Autodesk Inventor part; units mm, degrees
ref_plane "YZ Plane" through (0, 0, 0) normal (1, 0, 0) x (0, 1, 0)
ref_plane "XZ Plane" through (0, 0, 0) normal (0, 1, 0) x (-1, 0, 0)
ref_plane "XY Plane" through (0, 0, 0) normal (0, 0, 1) x (1, 0, 0)
sketch "Esboço1" plane through (0, 0, 0) normal (0, 1, 0) x (-1, 0, 0)
  arc A0 (-350, 0) -> (-247.4874, -247.4874) centre (0, 0) ccw
  arc A1 (-400, 0) -> (-282.8427, -282.8427) centre (0, 0) ccw
  circle A2 centre (0, 0) radius 400
  circle A3 centre (0, 0) radius 350
  line L0 (0, 0) -> (576.9105, 0)
  line L1 (0, 0) -> (-1224.3013, 0) construction
  line L2 (-350, 0) -> (-400, 0)
  point P0 (-282.8427, -282.8427)
  point P1 (-247.4874, -247.4874)
  point P2 (-282.8427, -282.8427)
  point P3 (400, 0)
  point P4 (350, 0)
  point P5 (-247.4874, -247.4874)
  dimension "d27" = 700
  dimension "d28" = 800
  dimension "d87" = 180
extrude "Extrusão1" add sketch "Esboço1" along normal blind 6 contours A0 A3 L0 A2 A1 L2
sketch "Esboço5" plane through (0, 6, 0) normal (0, 1, 0) x (1, 0, 0)
  arc A0 (400, 0) -> (-400, 0) centre (0, 0) ccw
  line L0 (-400, 0) -> (-350, 0)
  line L1 (0, 0) -> (-469.4096, 41.068)
  circle A1 centre (0, 0) radius 400
  arc A2 (350, 0) -> (-350, 0) centre (0, 0) ccw
  circle A3 centre (0, 0) radius 350
  line L2 (-400, 0) -> (-382, 0)
  line L3 (-382, 0) -> (-368, 0)
  line L4 (-398.4779, 34.8623) -> (-383.535, 33.555)
  line L5 (-383.535, 33.555) -> (-363.6111, 31.8118)
  line L6 (-382, 0) -> (-383.535, 33.555)
  line L7 (-368, 0) -> (-363.6111, 31.8118)
  point P0 (-348.6681, 30.5045)
  point P1 (-398.4779, 34.8623)
  point P2 (-348.6681, 30.5045)
  point P3 (-400, 0)
  dimension "d98" = -5
  dimension "d99" = 18
  dimension "d100" = 14
  dimension "d101" = 15
  dimension "d102" = 20
extrude "Extrusão5" cut sketch "Esboço5" against normal up to surface (6 mm away) contours L1 L7 L0 L6
sketch "Esboço6" plane through (0, 6, 0) normal (0, 1, 0) x (1, 0, 0)
  arc A0 (400, 0) -> (-400, 0) centre (0, 0) ccw
  circle A1 centre (0, 0) radius 400
  circle A2 centre (0, 0) radius 350
  line L0 (0, 0) -> (512.6153, -44.848)
  line L1 (350, 0) -> (400, 0)
  line L2 (350, 0) -> (368, 0)
  line L3 (368, 0) -> (382, 0)
  line L4 (382, 0) -> (400, 0)
  line L5 (348.6681, -30.5045) -> (363.6111, -31.8118)
  line L6 (363.6111, -31.8118) -> (383.535, -33.555)
  line L7 (383.535, -33.555) -> (398.4779, -34.8623)
  line L8 (368, 0) -> (363.6111, -31.8118)
  line L9 (382, 0) -> (383.535, -33.555)
  point P0 (-398.4779, 34.8623)
  dimension "d93" = 5
  dimension "d94" = 18
  dimension "d95" = 14
  dimension "d96" = 15
  dimension "d97" = 20
extrude "Extrusão6" add sketch "Esboço6" against normal up to surface (6 mm away) contours L9 L0 L8 L1
properties part number "base"
The listing builds one solid part. Answer for the finished solid, in the listing's coordinates (mm). Coordinates: 2 decimals unless noted, no trailing zeros. Loops run counter-clockwise (first coordinate to the right, second up) from the corner with the lowest first, then second, coordinate; pieces in that order, holes last. Notation, with made-up numbers: (11.5, -33) -> (45.5, -33) arc R9 ccw to (45.5, -26) -> close; hole circle Ø9 at (39, -15.75). An arc over 180 degrees is marked (long way). Return JSON: item names as keys, results as strings. Group by question number.
(1) A cutting plane is placed at D-D on x = 34.5. Write down the section's boundary in (y, z).
(2) A cutting plane is placed at C-C on y = 1.2. Write down the section's boundary in (x, z) (1 decimal).
(3) Find the intervals of material crossed by probe 1 along X at (y, z) = (3.75, -93.5); probe 2 along X at (y, z) = (1.1, -80); probe 3 along X at (y, z) = (1.55, 0.5), in increasing order. Write a range as from..to.
(4) A cutting plane is placed at B-B on z = -8.5. Write down the section's boundary in (x, y).
(5) A cutting plane is placed at A-A on z = -223.5. Write down the section's boundary in (x, y).
(6) Determine the mould class of faces 1 (the cylindrical face through (-159.147, 2.958, -366.977)), 2 (the flat face through (2, 6, -359)), 3 (the cylindrical face through (322.62, 2.96, -135.71)), 4 (the cylindrical face through (368.705, 2.958, -155.103)) for opening direction X: released by +X, released by -X, zero draft, split by the parting line, or undercut.
(7) Given pin 1 Ø3 at (x, y) = (-386.5, 1.5) entering from +Z; pin 2 Ø1.5 at (y, z) = (5, -290.5) entering from +X; pin 3 Ø5 at (x, z) = (308.5, -225.5) entering from -Y; pin 4 Ø1.5 at (y, z) = (3.5, -46) entering from +X, each flat-ended and moving along its own axis, determine where each tip first touches the part or whether it passes through.
The answers:
{
 "1": {"outline": "(0, -398.51) -> (6, -398.51) -> (6, -348.3) -> (0, -348.3) -> close"},
 "2": {"outline": "(-400, 0) arc R400 ccw to (282.8, -282.8) arc R400 ccw to (400, 0) -> (382, 0) -> (383.5, 33.6) -> (363.6, 31.8) -> (368, 0) -> (350, 0) arc R350 cw to (247.5, -247.5) arc R350 cw to (-350, 0) -> (-368, 0) -> (-363.6, -31.8) -> (-383.5, -33.6) -> (-382, 0) -> close"},
 "3": {"probe 1": "x = -388.92..-337.28, 337.28..388.92", "probe 2": "x = -391.92..-340.73, 340.73..391.92", "probe 3": "x = 367.93..382.02"},
 "4": {"outline": "(-399.91, 0) -> (-382.39, 0) -> (-382.39, 6) -> (-399.91, 6) -> close; (-366.83, 0) -> (-349.9, 0) -> (-349.9, 6) -> (-366.83, 6) -> close; (349.9, 0) -> (399.91, 0) -> (399.91, 6) -> (349.9, 6) -> close"},
 "5": {"outline": "(-331.73, 0) -> (-269.35, 0) -> (-269.35, 6) -> (-331.73, 6) -> close; (269.35, 0) -> (331.73, 0) -> (331.73, 6) -> (269.35, 6) -> close"},
 "6": {"face 1": "split by the parting line", "face 2": "zero draft", "face 3": "undercut", "face 4": "released by +X"},
 "7": {"pin 1": "stops at z = 0", "pin 2": "stops at x = 275.76", "pin 3": "stops at y = 0", "pin 4": "stops at x = 397.43"}
}
